Could you check a few things on this drawing? It's one solid part, dimensions in mm from its lowest x, y, z. Round coordinates to 2 decimals unless told otherwise and drop trailing zeros. Loops run counter-clockwise (first coordinate to the right, second up) from the corner with the lowest first, then second, coordinate; pieces in that order, holes last. Notation, with made-up numbers: (42.5, -32.75) -> (51.5, -32.75) arc R29 ccw to (51.5, -9.75) -> close; hole circle Ø8 at (31.5, -21.5). An arc over 180 degrees is marked (long way). Use one line per item in the form item = value. Start each with the question number.
Item 1: If I drill on L1, parallel to X at y = 3, z = 12; L2, parallel to Z at x = 137, y = 1; L3, parallel to Z at x = 12, y = 0.95, over which ranges is the centre line in solid material (lowest first)? Write a range as [from, to].
Item 2: I'm going to push a flat-ended pin straight in: pin 1 Ø1.5 at (y, z) = (1.5, 9) entering from -X. Where does the tip first touch, or does it pass through?
Item 3: If we section it at A-A (y = 2.8): Write out the boundary of the cut face in (x, z).
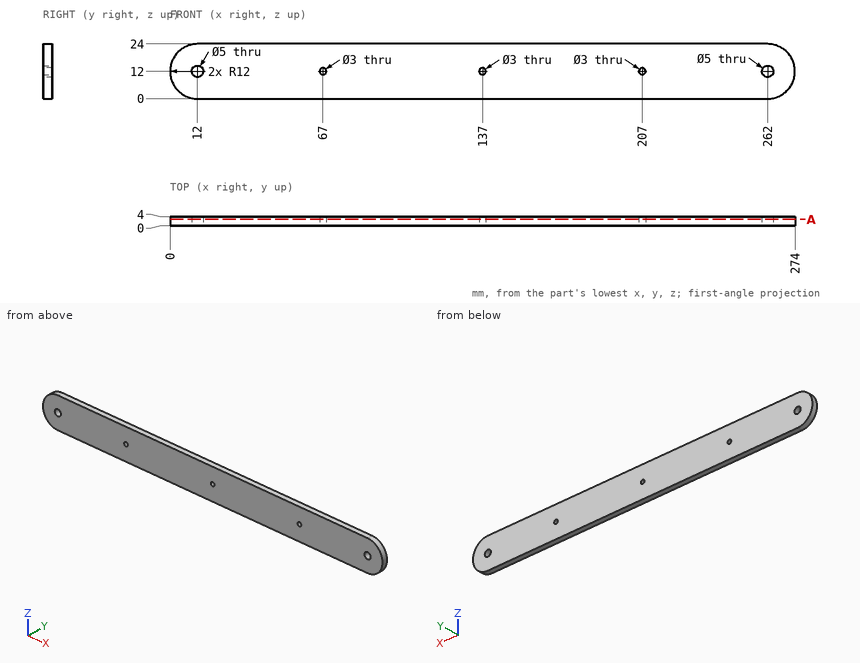
Values found:
q1.L1 = [0, 9.5], [14.5, 65.5], [68.5, 135.5], [138.5, 205.5], [208.5, 259.5], [264.5, 274]
q1.L2 = [0, 10.5], [13.5, 24]
q1.L3 = [0, 9.5], [14.5, 24]
q2.pin_1 = 0.21
q3.outline = (12, 0) -> (262, 0) arc R12 ccw to (262, 24) -> (12, 24) arc R12 ccw to start; hole circle Ø5 at (12, 12); hole circle Ø3 at (67, 12); hole circle Ø3 at (137, 12); hole circle Ø3 at (207, 12); hole circle Ø5 at (262, 12)
